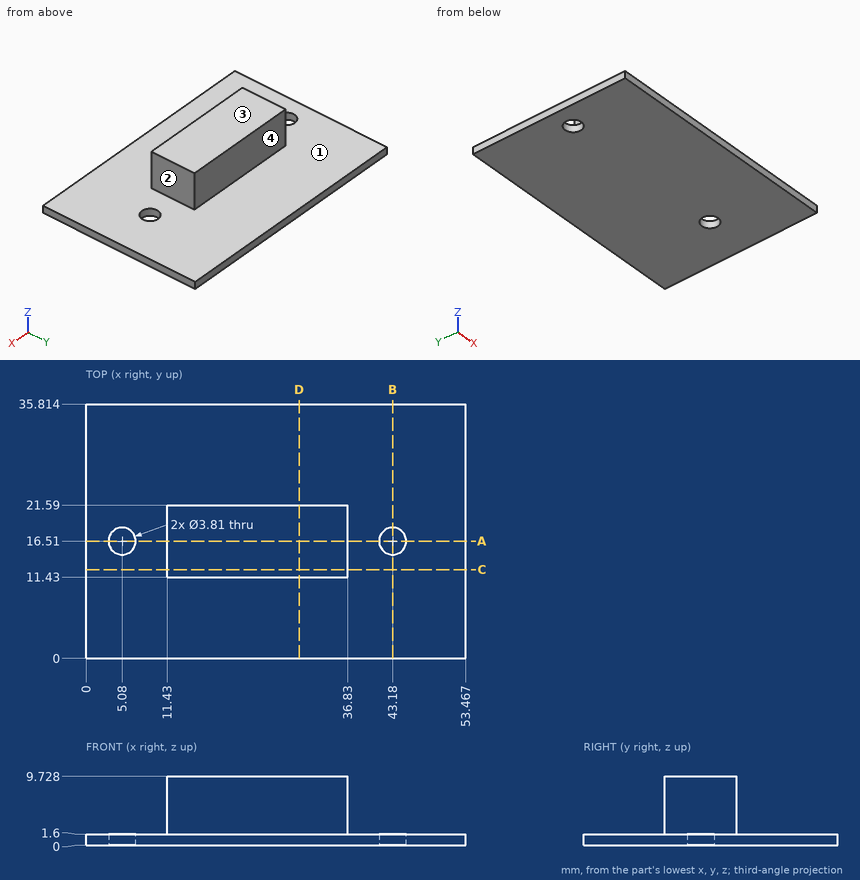
Geometry check sheet. Reference: drawing and pictorial views, mm from the part's lowest x, y, z. A direction names the side the tool comes from. Round coordinates to 2 decimals unless told otherwise and drop trailing zeros. Order: outer loops, then holes, each group sorted by start corner. A loop starts at its lowest first (then second) coordinate and runs counter-clockwise, first axis right, second up. Notation, with made-up numbers: M -9,-37.5 L -4,-37.5 A17 ccw -4,-24.5 Z; hole C 9.5,-20 d6. An arc over 180 degrees is marked long. Answer in a Markdown table with one row per item.
(1) Sectioned sample at B-B, the plane x = 43.18. Record the cut outline in (y, z) (1 decimal), and give its area (3 significant figures).
Responses:
| item | result |
|---|---|
| outline | M 0,0 L 14.6,0 L 14.6,1.6 L 0,1.6 Z; M 18.4,0 L 35.8,0 L 35.8,1.6 L 18.4,1.6 Z |
| area | 51.2 mm² |
(2) Sectioned sample at A-A, the plane y = 16.51. Record the cut outline in (x, z) (1 decimal).
Responses:
| item | result |
|---|---|
| outline | M 0,0 L 3.2,0 L 3.2,1.6 L 0,1.6 Z; M 7,0 L 41.3,0 L 41.3,1.6 L 36.8,1.6 L 36.8,9.7 L 11.4,9.7 L 11.4,1.6 L 7,1.6 Z; M 45.1,0 L 53.5,0 L 53.5,1.6 L 45.1,1.6 Z |
(3) Scan lines: probe 1 along Y at (x, z) = (43.18, 1) (3 decimals); probe 2 along X at (y, z) = (12.5, 7); probe 3 along Z at (x, y) = (42, 32.5). Record each from-to range of solid material in increasing order. Write a range as from..to.
Responses:
| item | result |
|---|---|
| probe 1 | y = 0..14.605, 18.415..35.814 |
| probe 2 | x = 11.43..36.83 |
| probe 3 | z = 0..1.6 |
(4) Sectioned sample at D-D, the plane x = 30. Record the cut outline in (y, z), and give its area (3 significant figures).
Responses:
| item | result |
|---|---|
| outline | M 0,0 L 35.81,0 L 35.81,1.6 L 21.59,1.6 L 21.59,9.73 L 11.43,9.73 L 11.43,1.6 L 0,1.6 Z |
| area | 140 mm² |
(5) Tool access check on the marked faces 3 and 4. Record the directions out of +Z, -Z, +X, -X, +Y, -Y that give a thin tool (end or side, any length) a straight path to the whole face; none if there is none.
Responses:
| item | result |
|---|---|
| face 3 | +Z, +X, -X, +Y, -Y |
| face 4 | +Z, +X, -X, +Y |
(6) Go/stop test with flat-tipped pins: P1, Ø4, axis at x = 28, z = 5.5, coming from the -Y side; P2, Ø2.5, axis at y = 18, z = 5.5, coming from the +X side; P3, Ø2.5, axis at x = 20, z = 7, coming from the +Y side. Record where each tip stops, or that it passes through.
Responses:
| item | result |
|---|---|
| P1 | stops at y = 11.43 |
| P2 | stops at x = 36.83 |
| P3 | stops at y = 21.59 |
(7) Sectioned sample at C-C, the plane y = 12.5. Record the cut outline in (x, z).
Responses:
| item | result |
|---|---|
| outline | M 0,0 L 53.47,0 L 53.47,1.6 L 36.83,1.6 L 36.83,9.73 L 11.43,9.73 L 11.43,1.6 L 0,1.6 Z |
(8) Draft check along X on the marked faces 1 and 2. Enter one of: released by +X, released by -X, zero draft, split by the parting line, or undercut.
Responses:
| item | result |
|---|---|
| face 1 | zero draft |
| face 2 | released by +X |
